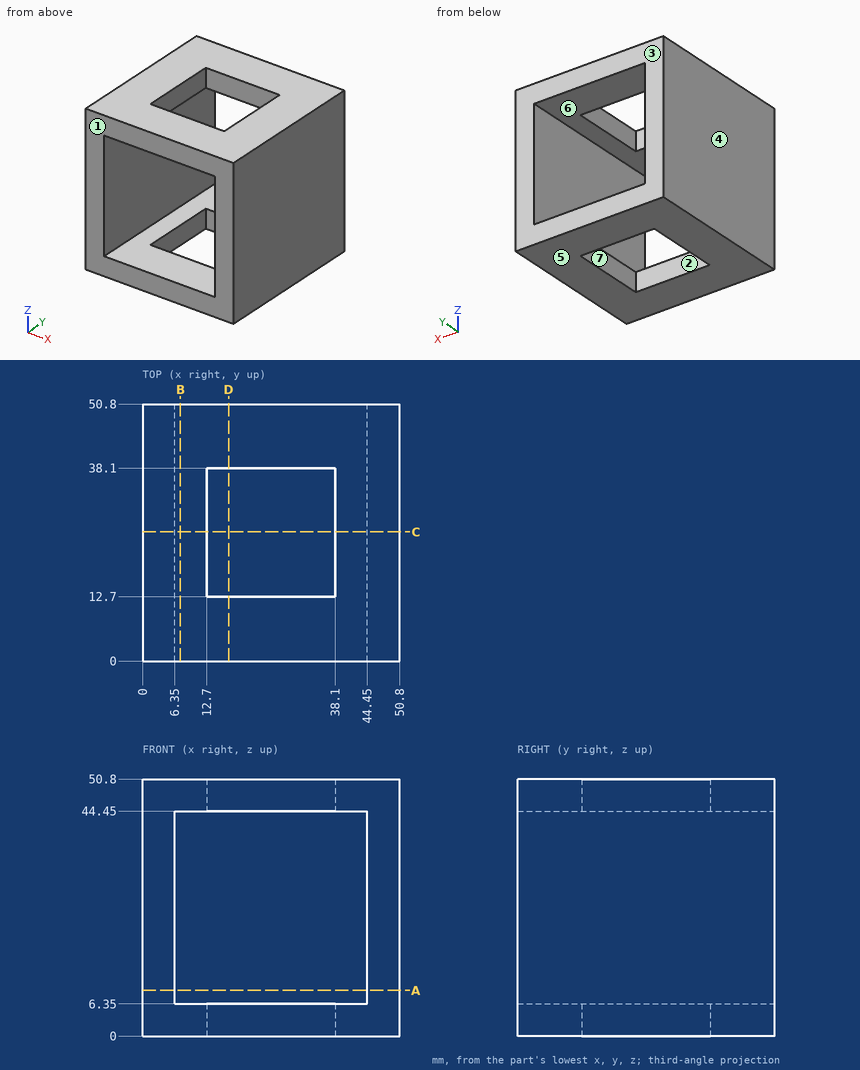
Source: three-view drawing plus pictorial views. Frame: mm from the lowest corner of the part. A direction names the side the tool comes from. Round coordinates to 2 decimals unless told otherwise and drop trailing zeros. Write each loop counter-clockwise with the first axis right and the second up, starting at its lowest first coordinate (ties: lowest second). Pieces come first, ordered by that corner, then holes. Notation, with made-up numbers: M 59.25,-21 L 113.25,-21 A16 cw 113.25,-1 Z; hole C -26.75,37 d11. An arc over 180 degrees is marked long. Write item = value, one per line.
Item 1: Section query B-B on x = 7.5. Return loops of the section in (y, z), then the cut area to 3 significant figures.
Findings:
outline = M 0,0 L 50.8,0 L 50.8,6.35 L 0,6.35 Z; M 0,44.45 L 50.8,44.45 L 50.8,50.8 L 0,50.8 Z
area = 645 mm^2
Item 2: Section query C-C on y = 25.5. Return loops of the section in (x, z), then the cut area to 3 significant figures.
Findings:
outline = M 0,0 L 12.7,0 L 12.7,6.35 L 6.35,6.35 L 6.35,44.45 L 12.7,44.45 L 12.7,50.8 L 0,50.8 Z; M 38.1,0 L 50.8,0 L 50.8,50.8 L 38.1,50.8 L 38.1,44.45 L 44.45,44.45 L 44.45,6.35 L 38.1,6.35 Z
area = 806 mm^2
Item 3: Section query A-A on z = 9. Return loops of the section in (x, y).
Findings:
outline = M 0,0 L 6.35,0 L 6.35,50.8 L 0,50.8 Z; M 44.45,0 L 50.8,0 L 50.8,50.8 L 44.45,50.8 Z
Item 4: Material intervals for line 1 along X through (y, z) = (17, 12); line 2 along Y through (x, z) = (14, 45), sorted ascending. Write a range as [from, to].
Findings:
line_1 = [0, 6.35], [44.45, 50.8]
line_2 = [0, 12.7], [38.1, 50.8]
Item 5: Pin query (flat end, axial travel): P1, Ø1.9, axis at y = 29.5, z = 47.5, coming from the -X side. Return the tip coordinate at first contact, or that it passes through.
Findings:
P1 = 0
Item 6: Section query D-D on x = 17. Return loops of the section in (y, z), then the cut area to 3 significant figures.
Findings:
outline = M 0,0 L 12.7,0 L 12.7,6.35 L 0,6.35 Z; M 0,44.45 L 12.7,44.45 L 12.7,50.8 L 0,50.8 Z; M 38.1,0 L 50.8,0 L 50.8,6.35 L 38.1,6.35 Z; M 38.1,44.45 L 50.8,44.45 L 50.8,50.8 L 38.1,50.8 Z
area = 323 mm^2
Item 7: Pull-direction query (Y, two-part tool) for the marked faces 1, 2, 3 and 4; classes: pulls with the +Y half, pulls with the -Y half, needs draft (parallel to the pull), parting line crosses it, or undercut.
Findings:
face_1 = pulls with the -Y half
face_2 = undercut
face_3 = pulls with the +Y half
face_4 = needs draft
Item 8: Access query for the marked faces 5, 6 and 7. Directions: +Z, -Z, +X, -X, +Y, -Y. A direction counts if a zero-diameter tool reaches every point of the face in a straight line with its end or side. Return the directions, or none.
Findings:
face_5 = -Z, +X, -X, +Y, -Y
face_6 = +Y, -Y
face_7 = +Z, -Z
